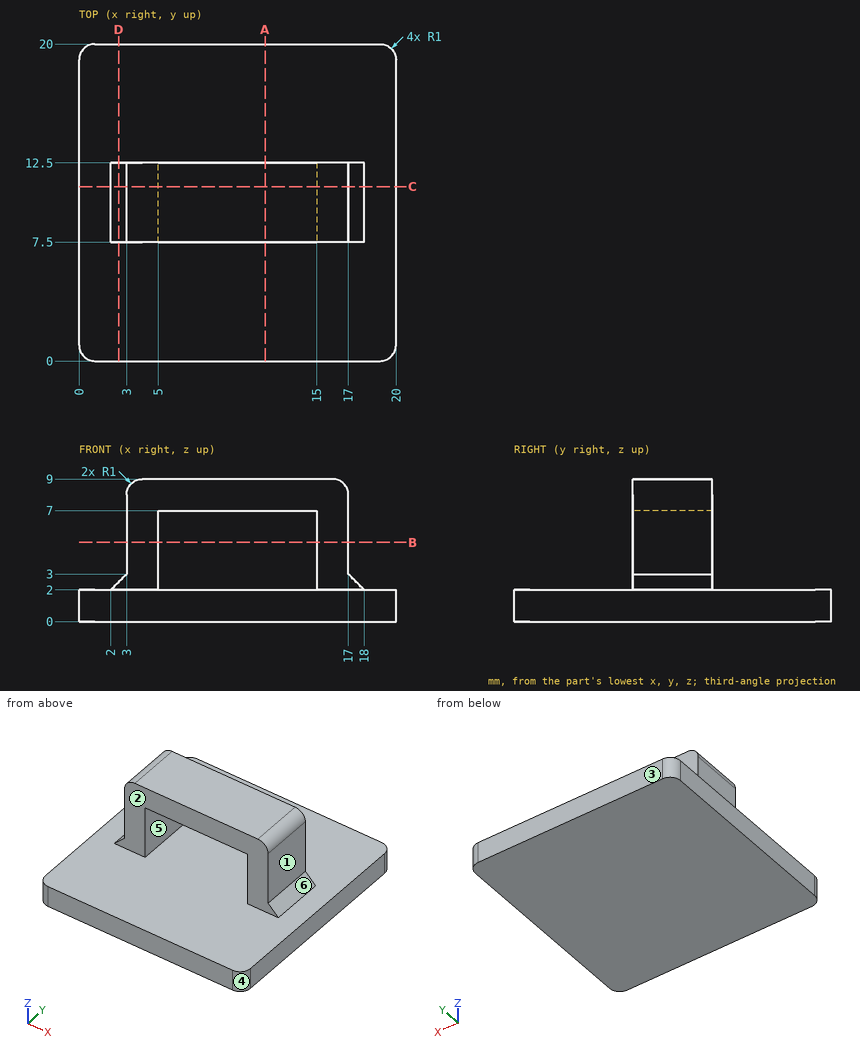
Design review of the part shown in the three views and the two pictorial views. Dimensions are in mm from the part's minimum x, y and z. A direction names the side the tool comes from. Round coordinates to 2 decimals unless told otherwise and drop trailing zeros. Loops run counter-clockwise (first coordinate to the right, second up) from the corner with the lowest first, then second, coordinate; pieces in that order, holes last. Notation, with made-up numbers: (0, 44) -> (39, 44) arc R17 ccw to (39, 65) -> close; hole circle Ø11 at (8.25, 54.25). An arc over 180 degrees is marked (long way). Return JSON: item names as keys, results as strings.
(1) Add section A-A on x = 11.75. Write out the cut boundary in (y, z).
Solved:
{"outline": "(0, 0) -> (20, 0) -> (20, 2) -> (0, 2) -> close; (7.5, 7) -> (12.5, 7) -> (12.5, 9) -> (7.5, 9) -> close"}
(2) For line 1 (X direction, y = 8.5, z = 4); line 2 (Y direction, x = 16, z = 7.25); line 3 (Z direction, x = 8.75, y = 4), list the stretches that pass through material, from the lowest coordinate up.
Solved:
{"line 1": "3 to 5, 15 to 17", "line 2": "7.5 to 12.5", "line 3": "0 to 2"}
(3) Add section B-B on z = 5. Write out the cut boundary in (x, y), plus the area to 3 significant figures.
Solved:
{"outline": "(3, 7.5) -> (5, 7.5) -> (5, 12.5) -> (3, 12.5) -> close; (15, 7.5) -> (17, 7.5) -> (17, 12.5) -> (15, 12.5) -> close", "area": "20.0 mm2"}
(4) For pin 1 (3 mm diameter, centred on y = 10.5, z = 4, fed in from -X); pin 2 (1.5 mm diameter, centred on y = 10, z = 4.5, fed in from +X); pin 3 (1.5 mm diameter, centred on y = 9.5, z = 4.5, fed in from -X), all flat-tipped, find the tip position at first contact; note any pin that passes through.
Solved:
{"pin 1": "x = 2.5", "pin 2": "x = 17", "pin 3": "x = 3"}
(5) Add section C-C on y = 11. Write out the cut boundary in (x, z), plus the area to 3 significant figures.
Solved:
{"outline": "(0, 0) -> (20, 0) -> (20, 2) -> (18, 2) -> (17, 3) -> (17, 8) arc R1 ccw to (16, 9) -> (4, 9) arc R1 ccw to (3, 8) -> (3, 3) -> (2, 2) -> (0, 2) -> close; hole (5, 2) -> (15, 2) -> (15, 7) -> (5, 7) -> close", "area": "88.6 mm2"}
(6) Add section D-D on x = 2.5. Write out the cut boundary in (y, z).
Solved:
{"outline": "(0, 0) -> (20, 0) -> (20, 2) -> (12.5, 2) -> (12.5, 2.5) -> (7.5, 2.5) -> (7.5, 2) -> (0, 2) -> close"}
(7) The part is to be moulded in two halves that separate along Z. For the marked faces 4, 5 and 6, say which applies: released by +Z, released by -Z, zero draft, split by the parting line, or undercut.
Solved:
{"face 4": "zero draft", "face 5": "undercut", "face 6": "released by +Z"}
(8) For the marked faces 1, 2 and 3, list the 3-axis set-ups (+Z, -Z, +X, -X, +Y, -Y) from which the entire face can be reached by the end or side of a thin tool; tool diameter is ignored.
Solved:
{"face 1": "+Z, +X, +Y, -Y", "face 2": "+Z, +X, -X, -Y", "face 3": "+Z, -Z, +X, -X, +Y"}
